Build history of the part. All positions in model axes, mm. Face numbers are marked on the shaded views. A direction names the side the tool comes from. Coordinates: 2 decimals unless noted, no trailing zeros. Loops run counter-clockwise (first coordinate to the right, second up) from the corner with the lowest first, then second, coordinate; pieces in that order, holes last.
(1) Slice it at C-C (x = -26). Give the cut face in (y, z), and give its area (3 significant figures).
(2) Tool access for the marked faces 4, 5, 6, 7 and 8: list every direction of +Z, -Z, +X, -X, +Y, -Y with a clear straight run to the whole face (end or side of a thin tool).
(3) Slice it at B-B (y = -42). Give the cut face in (x, z).
(4) Slice it at D-D (y = -18). Give the cut face in (x, z), and give its area (4 significant figures).
(5) Slice it at A-A (z = -7.5). Give the cut face in (x, y).
(6) Two-plate mould, pull along Z, no slides. Class the marked faces 1, 2 and 3: pulls with the +Z half, pulls with the -Z half, needs draft (parallel to the pull), parting line crosses it, or undercut.
(7) Wall check: L1, parallel to X at y = 44.2, z = 26; L2, parallel to Z at x = 0, y = 43.65; L3, parallel to X at y = -0.5, z = 27. Give the ranges that are in metal, low to high.
(8) Flat gauge pins, fed straight in: P1, Ø12.5, axis at x = -22, y = 22.5, coming from the +Z side; P2, Ø3, axis at y = -19, z = 1, coming from the -X side; P3, Ø1.2, axis at y = -1.5, z = 41.5, coming from the -X side. Where does each tip first touch, or does it go through?
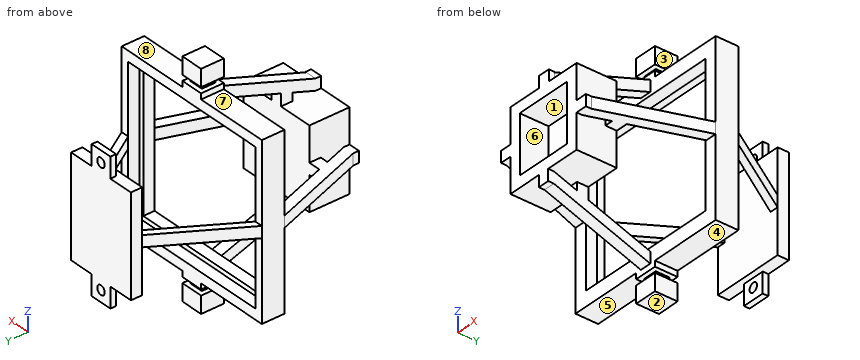
from build123d import *

# Parameters (mm, degrees)
SKETCH2_W                   = 75
SKETCH2_H                   = 75
BOSS_EXTRUDE1_DEPTH         = 5
SKETCH2_2_W                 = 75
SKETCH2_2_H                 = 75
BOSS_EXTRUDE2_DEPTH         = 5
SKETCH4_W                   = 68
SKETCH4_H                   = 66
CUT_EXTRUDE1_DEPTH          = 5
SKETCH5_W                   = 64
SKETCH5_H                   = 62
CUT_EXTRUDE2_DEPTH          = 5
SKETCH6_W                   = 10
SKETCH6_H                   = 10
BOSS_EXTRUDE3_DEPTH         = 2.5
SKETCH7_W                   = 6
SKETCH7_H                   = 6
BOSS_EXTRUDE4_DEPTH         = 2.5
SKETCH8_W                   = 10
SKETCH8_H                   = 10
BOSS_EXTRUDE5_DEPTH         = 7.5
SKETCH9_W                   = 10
SKETCH9_H                   = 10
BOSS_EXTRUDE6_DEPTH         = 2.5
SKETCH10_W                  = 6
SKETCH10_H                  = 6
BOSS_EXTRUDE7_DEPTH         = 2.5
SKETCH11_W                  = 10
SKETCH11_H                  = 10
BOSS_EXTRUDE8_DEPTH         = 7.5
SKETCH14_W                  = 35.4
SKETCH14_H                  = 35.4
BOSS_EXTRUDE9_DEPTH         = 17.7
SKETCH15_W                  = 25.4
SKETCH15_H                  = 25.4
CUT_EXTRUDE3_DEPTH          = 12.7
SKETCH32_R                  = 3
CUT_EXTRUDE6_DEPTH          = 5
SKETCH16_W                  = 32
SKETCH16_H                  = 44
BOSS_EXTRUDE10_DEPTH        = 5
SKETCH18_W                  = 10
SKETCH18_H                  = 9
BOSS_EXTRUDE12_DEPTH        = 2.5
BOSS_EXTRUDE13_DEPTH        = 2.5
BOSS_EXTRUDE14_DEPTH        = 2.5
SKETCH31_R                  = 2
CHARGER_SUPPORT_HOLES_DEPTH = 2.5
SKETCH27_W                  = 5
SKETCH27_H                  = 5
SKETCH27_W_2                = 5.344431893
EYEBOLT_BOLT_SUPPORTS_DEPTH = 2.5
BOSS_EXTRUDE15_DEPTH        = 2.5
BOSS_EXTRUDE16_DEPTH        = 2.5
BOSS_EXTRUDE17_DEPTH        = 2.5
BOSS_EXTRUDE18_DEPTH        = 2.5
SKETCH33_W                  = 6.3
SKETCH33_H                  = 5
SKETCH33_W_2                = 5
SKETCH33_H_2                = 6.3
EYEBOLT_MINI_SUPPORTS_DEPTH = 5


with BuildPart() as part:
    # Sketch2 → Boss-Extrude1 (new body)
    with BuildSketch(Plane(origin=(0, 0, 0), x_dir=(1, 0, 0), z_dir=(0, 1, 0))):
        Rectangle(SKETCH2_W, SKETCH2_H)
    extrude(amount=BOSS_EXTRUDE1_DEPTH)

    # Sketch2<2> → Boss-Extrude2 (add)
    with BuildSketch(Plane(origin=(0, 0, 0), x_dir=(1, 0, 0), z_dir=(0, 1, 0))):
        Rectangle(SKETCH2_2_W, SKETCH2_2_H)
    extrude(amount=-BOSS_EXTRUDE2_DEPTH)

    # Sketch4 → Cut-Extrude1 (cut)
    with BuildSketch(Plane(origin=(0, 5, 0), x_dir=(1, 0, 0), z_dir=(0, 1, 0))):
        Rectangle(SKETCH4_W, SKETCH4_H)
    extrude(amount=-CUT_EXTRUDE1_DEPTH, mode=Mode.SUBTRACT)

    # Sketch5 → Cut-Extrude2 (cut)
    with BuildSketch(Plane(origin=(0, 0, 0), x_dir=(1, 0, 0), z_dir=(0, 1, 0))):
        Rectangle(SKETCH5_W, SKETCH5_H)
    extrude(amount=-CUT_EXTRUDE2_DEPTH, mode=Mode.SUBTRACT)

    # Sketch6 → Boss-Extrude3 (add)
    with BuildSketch(Plane.XY.offset(37.5)):
        Rectangle(SKETCH6_W, SKETCH6_H)
    extrude(amount=BOSS_EXTRUDE3_DEPTH)

    # Sketch7 → Boss-Extrude4 (add)
    with BuildSketch(Plane.XY.offset(40)):
        Rectangle(SKETCH7_W, SKETCH7_H)
    extrude(amount=BOSS_EXTRUDE4_DEPTH)

    # Sketch8 → Boss-Extrude5 (add)
    with BuildSketch(Plane.XY.offset(42.5)):
        Rectangle(SKETCH8_W, SKETCH8_H)
    extrude(amount=BOSS_EXTRUDE5_DEPTH)

    # Sketch9 → Boss-Extrude6 (add)
    with BuildSketch(Plane(origin=(0, 0, -37.5), x_dir=(-1, 0, 0), z_dir=(0, 0, -1))):
        Rectangle(SKETCH9_W, SKETCH9_H)
    extrude(amount=BOSS_EXTRUDE6_DEPTH)

    # Sketch10 → Boss-Extrude7 (add)
    with BuildSketch(Plane(origin=(0, 0, -40), x_dir=(-1, 0, 0), z_dir=(0, 0, -1))):
        Rectangle(SKETCH10_W, SKETCH10_H)
    extrude(amount=BOSS_EXTRUDE7_DEPTH)

    # Sketch11 → Boss-Extrude8 (add)
    with BuildSketch(Plane(origin=(0, 0, -42.5), x_dir=(-1, 0, 0), z_dir=(0, 0, -1))):
        Rectangle(SKETCH11_W, SKETCH11_H)
    extrude(amount=BOSS_EXTRUDE8_DEPTH)



with BuildPart() as body_2:
    # Sketch14 → Boss-Extrude9 (new body)
    with BuildSketch(Plane(origin=(0, -50, 0), x_dir=(1, 0, 0), z_dir=(0, 1, 0))):
        Rectangle(SKETCH14_W, SKETCH14_H)
    extrude(amount=BOSS_EXTRUDE9_DEPTH)

    # Sketch15 → Cut-Extrude3 (cut)
    with BuildSketch(Plane.XZ.offset(50)):
        Rectangle(SKETCH15_W, SKETCH15_H)
    extrude(amount=-CUT_EXTRUDE3_DEPTH, mode=Mode.SUBTRACT)

    # Sketch32 → Cut-Extrude6 (cut)
    with BuildSketch(Plane(origin=(0, -32.3, 0), x_dir=(1, 0, 0), z_dir=(0, 1, 0))):
        Circle(SKETCH32_R)
    extrude(amount=-CUT_EXTRUDE6_DEPTH, mode=Mode.SUBTRACT)

    # Sketch27 → Eyebolt Bolt Supports (add)
    with BuildSketch(Plane(origin=(0, -50, 0), x_dir=(-1, 0, 0), z_dir=(0, -1, 0))):
        with Locations((-20.2, 0)):
            Rectangle(SKETCH27_W, SKETCH27_H)
        with Locations((20.2, 0)):
            Rectangle(SKETCH27_W, SKETCH27_H)
        with Locations((-0.172215947, -20.2)):
            Rectangle(SKETCH27_W_2, SKETCH27_H)
        with Locations((0, 20.2)):
            Rectangle(SKETCH27_W, SKETCH27_H)
    extrude(amount=-EYEBOLT_BOLT_SUPPORTS_DEPTH)


with BuildPart() as body_3:
    # Sketch16 → Boss-Extrude10 (new body)
    with BuildSketch(Plane(origin=(0, 45, 0), x_dir=(1, 0, 0), z_dir=(0, 1, 0))):
        Rectangle(SKETCH16_W, SKETCH16_H)
    extrude(amount=-BOSS_EXTRUDE10_DEPTH)

    # Sketch18 → Boss-Extrude12 (add)
    with BuildSketch(Plane(origin=(0, 45, 0), x_dir=(1, 0, 0), z_dir=(0, 1, 0))):
        with Locations((0, 26.5)):
            Rectangle(SKETCH18_W, SKETCH18_H)
        with Locations((0, -26.5)):
            Rectangle(SKETCH18_W, SKETCH18_H)
    extrude(amount=-BOSS_EXTRUDE12_DEPTH)


with BuildPart() as part_1:
    add(part.part)

    add(body_3.part)  # Boss-Extrude13 merges body 3
    # Sketch21 → Boss-Extrude13 (add)
    with BuildSketch(Plane.XY):
        Polygon((-37.5, 5), (-34, 5), (-12.434815796, 40), (-16, 40), align=None)
        Polygon((37.5, 5), (34, 5), (12.245590879, 40), (16, 40), align=None)
    extrude(amount=BOSS_EXTRUDE13_DEPTH)

    # Sketch21<2> → Boss-Extrude14 (add)
    with BuildSketch(Plane.XY):
        Polygon((-37.5, 5), (-34, 5), (-12.434815796, 40), (-16, 40), align=None)
        Polygon((37.5, 5), (34, 5), (12.245590879, 40), (16, 40), align=None)
    extrude(amount=-BOSS_EXTRUDE14_DEPTH)

    # Sketch31 → Charger Support Holes (cut)
    with BuildSketch(Plane(origin=(0, 45, 0), x_dir=(1, 0, 0), z_dir=(0, 1, 0))):
        with Locations((0, 26)):
            Circle(SKETCH31_R)
        with Locations((0, -26)):
            Circle(SKETCH31_R)
    extrude(amount=-CHARGER_SUPPORT_HOLES_DEPTH, mode=Mode.SUBTRACT)


    add(body_2.part)  # Boss-Extrude15 merges body 2
    # Sketch28 → Boss-Extrude15 (add)
    with BuildSketch(Plane.XY):
        Polygon((22.7, -47.5), (37.5, -5), (32.5, -5), (17.7, -47.5), align=None)
        Polygon((-22.7, -47.5), (-37.5, -5), (-32.5, -5), (-17.7, -47.5), align=None)
    extrude(amount=BOSS_EXTRUDE15_DEPTH)

    # Sketch28<2> → Boss-Extrude16 (add)
    with BuildSketch(Plane.XY):
        Polygon((22.7, -47.5), (37.5, -5), (32.5, -5), (17.7, -47.5), align=None)
        Polygon((-22.7, -47.5), (-37.5, -5), (-32.5, -5), (-17.7, -47.5), align=None)
    extrude(amount=-BOSS_EXTRUDE16_DEPTH)

    # Sketch30 → Boss-Extrude17 (add)
    with BuildSketch(Plane(origin=(0, 0, 0), x_dir=(0, 0, -1), z_dir=(1, 0, 0))):
        Polygon((22.7, -47.5), (37.5, -5), (32.5, -5), (17.7, -47.5), align=None)
        Polygon((-37.5, -5), (-22.7, -47.5), (-17.7, -47.5), (-32.5, -5), align=None)
    extrude(amount=BOSS_EXTRUDE17_DEPTH)

    # Sketch30<2> → Boss-Extrude18 (add)
    with BuildSketch(Plane(origin=(0, 0, 0), x_dir=(0, 0, -1), z_dir=(1, 0, 0))):
        Polygon((22.7, -47.5), (37.5, -5), (32.5, -5), (17.7, -47.5), align=None)
        Polygon((-37.5, -5), (-22.7, -47.5), (-17.7, -47.5), (-32.5, -5), align=None)
    extrude(amount=-BOSS_EXTRUDE18_DEPTH)

    # Sketch33 → Eyebolt Mini Supports (add)
    with BuildSketch(Plane(origin=(0, -32.3, 0), x_dir=(1, 0, 0), z_dir=(0, 1, 0))):
        with Locations((20.85, 0)):
            Rectangle(SKETCH33_W, SKETCH33_H)
        with Locations((0, 20.85)):
            Rectangle(SKETCH33_W_2, SKETCH33_H_2)
        with Locations((-20.85, 0)):
            Rectangle(SKETCH33_W, SKETCH33_H)
        with Locations((0, -20.85)):
            Rectangle(SKETCH33_W_2, SKETCH33_H_2)
    extrude(amount=-EYEBOLT_MINI_SUPPORTS_DEPTH)


solid = part_1.part
Response values:
1. outline: (-38.02, -2.5) - (-23.67, -2.5) - (-23.67, 2.5) - (-38.02, 2.5) - close; (-5, -37.5) - (5, -37.5) - (5, -33) - (0, -33) - (0, -31) - (-5, -31) - close; (-5, 31) - (0, 31) - (0, 33) - (5, 33) - (5, 37.5) - (-5, 37.5) - close; (17.98, -2.5) - (23.72, -2.5) - (23.72, 2.5) - (17.98, 2.5) - close
1. area: 210 mm2
2. face 4: -Z, +X, +Y, -Y
2. face 5: -Z, -X, +Y, -Y
2. face 6: -Y
2. face 7: +Z, -X, +Y, -Y
2. face 8: +Z, +X, +Y, -Y
3. outline: (-24.62, -2.5) - (-19.62, -2.5) - (-19.62, 2.5) - (-24.62, 2.5) - close; (-17.7, -17.7) - (17.7, -17.7) - (17.7, 17.7) - (-17.7, 17.7) - close; (-2.5, -24.62) - (2.5, -24.62) - (2.5, -19.62) - (-2.5, -19.62) - close; (-2.5, 19.62) - (2.5, 19.62) - (2.5, 24.62) - (-2.5, 24.62) - close; (19.62, -2.5) - (24.62, -2.5) - (24.62, 2.5) - (19.62, 2.5) - close; hole (-12.7, -12.7) - (12.7, -12.7) - (12.7, 12.7) - (-12.7, 12.7) - close
4. outline: (-32.97, -2.5) - (-27.97, -2.5) - (-27.97, 2.5) - (-32.97, 2.5) - close; (-2.5, -32.97) - (2.5, -32.97) - (2.5, -27.97) - (-2.5, -27.97) - close; (-2.5, 27.97) - (2.5, 27.97) - (2.5, 32.97) - (-2.5, 32.97) - close; (27.97, -2.5) - (32.97, -2.5) - (32.97, 2.5) - (27.97, 2.5) - close
4. area: 100.0 mm2
5. outline: (-37.5, -5) - (-32, -5) - (-32, 0) - (-34, 0) - (-34, 5) - (-37.5, 5) - close; (-17.7, -50) - (-12.7, -50) - (-12.7, -37.3) - (12.7, -37.3) - (12.7, -50) - (17.7, -50) - (17.7, -32.3) - (-17.7, -32.3) - close; (-16, 40) - (16, 40) - (16, 45) - (-16, 45) - close; (32, -5) - (37.5, -5) - (37.5, 5) - (34, 5) - (34, 0) - (32, 0) - close
6. face 1: undercut
6. face 2: pulls with the -Z half
6. face 3: needs draft
7. L1: x = -5 to -2, 2 to 5
7. L2: z = -31 to -28, -24 to 24, 28 to 31
7. L3: x = -37.5 to -32, 32 to 37.5
8. P1: stops at z = 2.5
8. P2: stops at x = -33.15
8. P3: stops at x = -3
